```python
from build123d import *

# Parameters (mm, degrees)
SKETCH1_W               = 7.1
SKETCH1_H               = 5.6
BOSS_EXTRUDE1_DEPTH     = 3.35
SKETCH2_W               = 4
SKETCH2_H               = 4
BOSS_EXTRUDE2_DEPTH     = 3.5
SKETCH3_W               = 1.45
SKETCH3_H               = 1.45
CUT_EXTRUDE1_DEPTH      = 3.5
MIRROR2_COPY_1_SKETCH_W = 1.45
MIRROR2_COPY_1_SKETCH_H = 1.45
MIRROR2_COPY_1_DEPTH    = 3.5
SKETCH4_W               = 5
SKETCH4_H               = 2.2
BOSS_EXTRUDE3_DEPTH     = 0.75
SKETCH5_W               = 5.5
SKETCH5_H               = 5.6
CUT_EXTRUDE2_DEPTH      = 3
SKETCH6_R               = 2.4
CUT_EXTRUDE3_DEPTH      = 2
SKETCH7_R               = 1
BOSS_EXTRUDE4_DEPTH     = 7.3
CHAMFER1_SIZE           = 0.5
BOSS_EXTRUDE5_DEPTH     = 0.8
SKETCH9_R               = 0.4
CUT_EXTRUDE4_DEPTH      = 0.8


with BuildPart() as part:
    # Sketch1 → Boss-Extrude1 (new, symmetric)
    with BuildSketch(Plane.XY):
        Rectangle(SKETCH1_W, SKETCH1_H)
    extrude(amount=BOSS_EXTRUDE1_DEPTH, both=True)

    # Sketch2 → Boss-Extrude2 (add)
    with BuildSketch(Plane.XY.offset(3.35)):
        Rectangle(SKETCH2_W, SKETCH2_H)
    extrude(amount=BOSS_EXTRUDE2_DEPTH)

    # Sketch3 → Cut-Extrude1 (cut)
    with BuildSketch(Plane.XY.offset(6.85)):
        with Locations((-1.275, 1.275)):
            Rectangle(SKETCH3_W, SKETCH3_H)
    cut_extrude1 = extrude(amount=-CUT_EXTRUDE1_DEPTH, mode=Mode.SUBTRACT)

    # Mirror1: Cut-Extrude1 across plane
    add(cut_extrude1.mirror(Plane(origin=(0, 0, 0), x_dir=(0, 0, 1), z_dir=(1, 0, 0))), mode=Mode.SUBTRACT)

    # Mirror2: Cut-Extrude1 across plane
    add(cut_extrude1.mirror(Plane.ZX), mode=Mode.SUBTRACT)

    # Mirror2 copy 1 sketch → Mirror2 copy 1 (cut)
    with BuildSketch(Plane(origin=(0, 0, 6.85), x_dir=(-1, 0, 0), z_dir=(0, 0, 1))):
        with Locations((-1.275, 1.275)):
            Rectangle(MIRROR2_COPY_1_SKETCH_W, MIRROR2_COPY_1_SKETCH_H)
    extrude(amount=-MIRROR2_COPY_1_DEPTH, mode=Mode.SUBTRACT)

    # Sketch4 → Boss-Extrude3 (add)
    with BuildSketch(Plane.ZY.offset(3.55)):
        with Locations((-0.85, 0)):
            Rectangle(SKETCH4_W, SKETCH4_H)
    boss_extrude3 = extrude(amount=BOSS_EXTRUDE3_DEPTH)

    # Mirror3: Boss-Extrude3 across plane
    add(boss_extrude3.mirror(Plane(origin=(0, 0, 0), x_dir=(0, 0, 1), z_dir=(1, 0, 0))))

    # Sketch5 → Cut-Extrude2 (cut)
    with BuildSketch(Plane(origin=(0, 0, -3.35), x_dir=(-1, 0, 0), z_dir=(0, 0, -1))):
        Rectangle(SKETCH5_W, SKETCH5_H)
    extrude(amount=-CUT_EXTRUDE2_DEPTH, mode=Mode.SUBTRACT)

    # Sketch6 → Cut-Extrude3 (cut)
    with BuildSketch(Plane(origin=(0, 0, -0.35), x_dir=(-1, 0, 0), z_dir=(0, 0, -1))):
        Circle(SKETCH6_R)
    extrude(amount=-CUT_EXTRUDE3_DEPTH, mode=Mode.SUBTRACT)

    # Sketch7 → Boss-Extrude4 (add)
    with BuildSketch(Plane(origin=(0, 0, 1.65), x_dir=(-1, 0, 0), z_dir=(0, 0, -1))):
        Circle(SKETCH7_R)
    extrude(amount=BOSS_EXTRUDE4_DEPTH)

    # Chamfer1
    chamfer1_edges = [part.edges().sort_by_distance(p)[0] for p in [
        (1, 0, -5.65),
    ]]
    chamfer(chamfer1_edges, length=CHAMFER1_SIZE)

    # Sketch8 → Boss-Extrude5 (add)
    with BuildSketch(Plane(origin=(3.55, 0, 0), x_dir=(0, 0, -1), z_dir=(1, 0, 0))):
        Polygon((1.35, -2.8), (2.35, -3.8), (3.35, -3.8), (3.35, -2.8), align=None)
    boss_extrude5 = extrude(amount=-BOSS_EXTRUDE5_DEPTH)

    # Sketch9 → Cut-Extrude4 (cut)
    with BuildSketch(Plane(origin=(3.55, 0, 0), x_dir=(0, 0, -1), z_dir=(1, 0, 0))):
        with Locations((3.35, -3.2)):
            Circle(SKETCH9_R)
    cut_extrude4 = extrude(amount=-CUT_EXTRUDE4_DEPTH, mode=Mode.SUBTRACT)

    # Mirror4: Boss-Extrude5, Cut-Extrude4 across plane
    add(boss_extrude5.mirror(Plane(origin=(0, 0, 0), x_dir=(0, 0, 1), z_dir=(1, 0, 0))))
    add(cut_extrude4.mirror(Plane(origin=(0, 0, 0), x_dir=(0, 0, 1), z_dir=(1, 0, 0))), mode=Mode.SUBTRACT)


solid = part.part
```
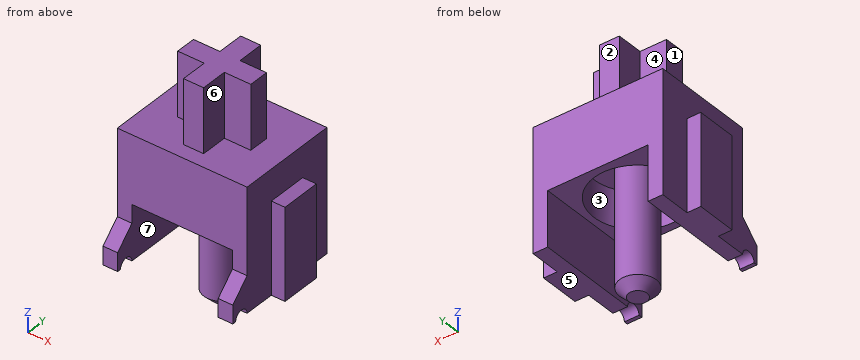
The listing builds one solid part. Answer for the finished solid, in the listing's coordinates (mm). Face numbers are marked on the shaded views. A direction names the side the tool comes from. Give positions to 0.01 mm unless a question says otherwise; leave off trailing zeros. Order: outer loops, then holes, each group sorted by start corner. A loop starts at its lowest first (then second) coordinate and runs counter-clockwise, first axis right, second up.
1) Given P1, Ø1.5, axis at x = 0.5, z = -4, coming from the +Y side; P2, Ø0.8, axis at x = 3.5, y = 0.5, coming from the -Z side; P3, Ø0.6, axis at x = -4, z = 0, coming from the -Y side, each flat-ended and moving along its own axis, determine where each tip first touches the part or whether it passes through.
Reported:
P1: stops at y = 1
P2: stops at z = -3.35
P3: stops at y = -1.1
2) Find section D-D on x = 0. Write down the section's boundary in (y, z), then the cut area to 3 significant figures.
Reported:
outline: (-2.8, -0.35) - (-2.4, -0.35) - (-2.4, 1.65) - (-1, 1.65) - (-1, -5.15) - (-0.5, -5.65) - (0.5, -5.65) - (1, -5.15) - (1, 1.65) - (2.4, 1.65) - (2.4, -0.35) - (2.8, -0.35) - (2.8, 3.35) - (2, 3.35) - (2, 6.85) - (-2, 6.85) - (-2, 3.35) - (-2.8, 3.35) - close
area: 39.5 mm2
3) Consider line 1 along Y through (x, z) = (0, 0.8); line 2 along X through (y, z) = (-2.5, -2.75); line 3 along Z through (x, y) = (-1, -1.25). Determine where each line is inside the solid, lowest interval first.
Reported:
line 1: y = -2.8 to -2.4, -1 to 1, 2.4 to 2.8
line 2: x = -3.55 to -2.75, 2.75 to 3.55
line 3: z = 1.65 to 3.35
4) Find section A-A on z = -2. Write down the section's boundary in (x, y).
Reported:
outline: (-4.3, -1.1) - (-3.55, -1.1) - (-3.55, -3.45) - (-2.75, -3.45) - (-2.75, 2.8) - (-3.55, 2.8) - (-3.55, 1.1) - (-4.3, 1.1) - close; circle Ø2 at (0, 0); (2.75, -3.45) - (3.55, -3.45) - (3.55, -1.1) - (4.3, -1.1) - (4.3, 1.1) - (3.55, 1.1) - (3.55, 2.8) - (2.75, 2.8) - close
5) Determine the mould class of the marked faces 1, 2 and 3 for opening direction X: pulls with the +X half, pulls with the -X half, needs draft (parallel to the pull), parting line crosses it, or undercut.
Reported:
face 1: pulls with the -X half
face 2: needs draft
face 3: undercut
6) Find section C-C on y = -3.2. Write down the section's boundary in (x, z).
Reported:
outline: (-3.55, -2.95) - (-2.75, -2.95) - (-2.75, -1.75) - (-3.55, -1.75) - close; (2.75, -2.95) - (3.55, -2.95) - (3.55, -1.75) - (2.75, -1.75) - close
7) Find section B-B on z = 0. Write down the section's boundary in (x, y).
Reported:
outline: (-4.3, -1.1) - (-3.55, -1.1) - (-3.55, -2.8) - (3.55, -2.8) - (3.55, -1.1) - (4.3, -1.1) - (4.3, 1.1) - (3.55, 1.1) - (3.55, 2.8) - (-3.55, 2.8) - (-3.55, 1.1) - (-4.3, 1.1) - close; circle Ø2 at (0, 0); hole circle Ø4.8 at (0, 0)
8) For the marked faces 4, 5, 6 and 7, determine the directions among +Z, -Z, +X, -X, +Y, -Y from which every point of the face is accessible in a straight line to the end or side of a thin tool.
Reported:
face 4: +Z, -X, +Y
face 5: -Z, +X, +Y, -Y
face 6: +Z, +X, -Y
face 7: -Z, +Y, -Y
